The model under review builds one solid part; all positions refer to its coordinate system, in mm. Coordinates: 2 decimals unless noted, no trailing zeros. Write each loop counter-clockwise with the first axis right and the second up, starting at its lowest first coordinate (ties: lowest second). Pieces come first, ordered by that corner, then holes.
Autodesk Inventor part; units mm, degrees
ref_plane "YZ Plane" through (0, 0, 0) normal (1, 0, 0) x (0, 1, 0)
ref_plane "XZ Plane" through (0, 0, 0) normal (0, 1, 0) x (-1, 0, 0)
ref_plane "XY Plane" through (0, 0, 0) normal (0, 0, 1) x (1, 0, 0)
sketch "Key" plane through (0, 0, 0) normal (0, 0, 1) x (1, 0, 0)
  line L0 (-9.525, 9.525) -> (9.525, 9.525) construction
  line L1 (9.525, 9.525) -> (9.525, -9.525) construction
  line L2 (9.525, -9.525) -> (-9.525, -9.525) construction
  line L3 (-9.525, -9.525) -> (-9.525, 9.525) construction
  line L4 (-9.525, 9.525) -> (9.525, -9.525) construction
  line L5 (9.525, 9.525) -> (-9.525, -9.525) construction
  point P0 (0, 0)
  point P1 (0, 0)
  dimension "d6" = 19.05
  dimension "d7" = 19.05
sketch "Col5" plane through (0, 0, 0) normal (0, 0, 1) x (1, 0, 0)
  point P0 (-10.8651, 0)
sketch "Col4" plane through (0, 0, 0) normal (0, 0, 1) x (1, 0, 0)
  point P0 (-10.8651, 0)
sketch "TC" plane through (0, 0, 0) normal (0, 0, 1) x (1, 0, 0)
  point P0 (-22.1335, 152.0917)
  dimension "d12" = 4.7625
  dimension "d13" = 4.7625
  dimension "d14" = 19.6363
sketch "Esquisse1" plane through (0, 0, 0) normal (1, 0, 0) x (0, 1, 0)
  line L0 (28.177, -71.755) -> (10.397, -71.755) construction
  line L1 (10.397, -71.755) -> (10.397, -102.235) construction
  line L2 (10.397, -102.235) -> (28.177, -102.235)
  line L3 (28.177, -102.235) -> (28.177, -71.755) construction
  line L4 (28.177, -71.755) -> (10.397, -102.235) construction
  line L5 (10.397, -71.755) -> (28.177, -102.235) construction
  line L6 (6.445, 14.065) -> (-92.805, 14.065)
  line L7 (6.445, 14.065) -> (6.445, -24.035)
  line L8 (-68.4861, -104.235) -> (30.177, -104.235)
  line L9 (30.177, -51.755) -> (30.177, -104.235)
  line L10 (-106.1694, -150.4545) -> (-142.6291, -129.4045)
  line L11 (-103.8052, -81.2096) -> (-113.3302, -97.7073)
  line L12 (-113.3302, -97.7073) -> (-117.4547, -95.3261)
  line L13 (-117.4547, -95.3261) -> (-126.9797, -111.8239)
  line L14 (-126.9797, -111.8239) -> (-131.1041, -109.4426)
  line L15 (-131.1041, -109.4426) -> (-142.6291, -129.4045)
  line L16 (-68.4861, -104.235) -> (-78.8706, -122.2214)
  line L17 (-78.8706, -122.2214) -> (-82.995, -119.8402)
  line L18 (-82.995, -119.8402) -> (-92.52, -136.338)
  line L19 (-92.52, -136.338) -> (-96.6444, -133.9567)
  line L20 (-96.6444, -133.9567) -> (-106.1694, -150.4545)
  line L21 (-92.805, 14.065) -> (-92.805, -28.035)
  line L22 (-92.805, -28.035) -> (-88.042, -28.035)
  line L23 (-88.042, -28.035) -> (-88.042, -47.085)
  line L24 (-88.042, -47.085) -> (-85.565, -47.085)
  line L25 (-85.565, -47.085) -> (-85.565, -62.135)
  line L26 (-85.565, -62.135) -> (-87.565, -62.135)
  line L27 (-89.5164, -89.4592) -> (-103.8052, -81.2096) construction
  line L28 (6.445, -24.035) -> (11.208, -24.035)
  line L29 (11.208, -24.035) -> (11.208, -43.085)
  line L30 (11.208, -43.085) -> (13.685, -43.085)
  line L31 (30.177, -51.755) -> (13.685, -43.085)
  line L32 (-78.8706, -122.2214) -> (-92.52, -136.338) construction
  line L33 (-92.52, -136.338) -> (-106.1694, -150.4545) construction
  line L34 (-103.8052, -81.2096) -> (-117.4547, -95.3261) construction
  line L35 (-131.1041, -109.4426) -> (-117.4547, -95.3261) construction
  line L36 (-103.8052, -81.2096) -> (-87.565, -81.2096)
  line L37 (-87.565, -81.2096) -> (-87.565, -62.135)
  point P0 (-5.08, 2.54)
  point P1 (19.287, -86.995)
  point P2 (-5.08, 2.54)
  point P3 (-86.042, -35.56)
  point P4 (0, 0)
extrude "Extrusion1" add sketch "Esquisse1" along normal blind 1.6
chamfer "Chanfrein5" distance 1 angle 45 6 edges at (0.8, -117.4547, -95.3261) (0.8, -131.1041, -109.4426) (0.8, -142.6291, -129.4045) (0.8, -106.1694, -150.4545) (0.8, -92.52, -136.338) (0.8, -78.8706, -122.2214)
properties part number "board-profile"
Item 1: Mouldability with a two-part tool opening along Y and no side actions: class faces 1 (the face through (1.6, -38, -67)), 2 (the face through (0.789, -124.156, -140.07)), 3 (the face through (0.79, -73.36, -112.68)) as pulls with the +Y half, pulls with the -Y half, needs draft (parallel to the pull), parting line crosses it, or undercut.
Solved:
face 1: needs draft
face 2: pulls with the -Y half
face 3: pulls with the +Y half
Item 2: Take a section at B-B, the plane y = -31. Write out the cut boundary in (x, z) (3 decimals).
Solved:
outline: (0, -104.235) - (1.6, -104.235) - (1.6, 14.065) - (0, 14.065) - close
Item 3: Take a section at C-C, the plane z = -14.5. Write out the cut boundary in (x, y) (3 decimals), plus the area to 3 significant figures.
Solved:
outline: (0, -92.805) - (1.6, -92.805) - (1.6, 6.445) - (0, 6.445) - close
area: 159 mm2
Item 4: For pin 1 (0.8 mm diameter, centred on x = 1, y = -86.5, fed in from -Z); pin 2 (0.5 mm diameter, centred on x = 1, y = -28, fed in from -Z) (3 decimals); pin 3 (0.5 mm diameter, centred on x = 0.5, z = -51.5, fed in from -Y) (3 decimals), all flat-tipped, find the tip position at first contact; note any pin that passes through.
Solved:
pin 1: stops at z = -126.6
pin 2: stops at z = -104.235
pin 3: stops at y = -85.565
Item 5: To check wall thickness, follow line 1 along Y through (x, z) = (1.3, -84.5); line 2 along Y through (x, z) = (0.9, -79.5) (3 decimals); line 3 along Z through (x, y) = (0.85, -11) (3 decimals). State the ranges of each line that lie inside material, in increasing order.
Solved:
line 1: y = -105.7 to 30.18
line 2: y = -87.565 to 30.177
line 3: z = -104.235 to 14.065
